Input: part model. Units: mm. Frame: model coordinates. Face numbers are marked on the shaded views. A direction names the side the tool comes from. Coordinates: 2 decimals unless noted, no trailing zeros. Loops run counter-clockwise (first coordinate to the right, second up) from the corner with the lowest first, then second, coordinate; pieces in that order, holes last. Notation, with made-up numbers: (-37.75, -30) -> (5.25, -30) arc R7 ccw to (5.25, -23) -> close; hole circle Ø2 at (53, 32). An arc over 180 degrees is marked (long way). Answer as a JSON object with one key per item and string values.
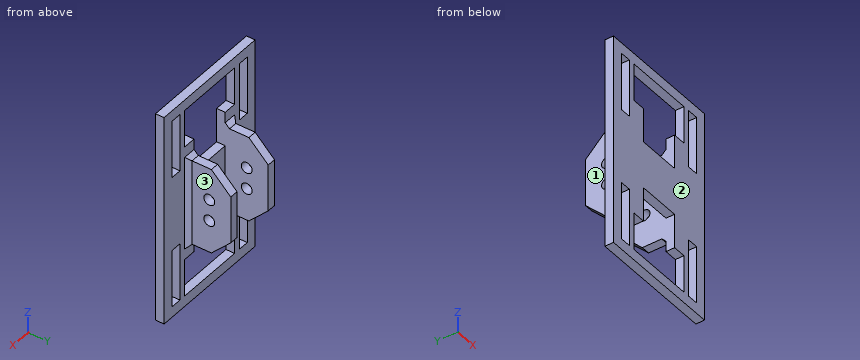
from build123d import *

# Parameters (mm, degrees)
SKETCH1_W           = 58.28
SKETCH1_H           = 99
SKETCH1_W_2         = 5.14
SKETCH1_H_2         = 27
BOSS_EXTRUDE1_DEPTH = 4
SKETCH2_W           = 4
SKETCH2_H           = 40
BOSS_EXTRUDE2_DEPTH = 20
CUT_EXTRUDE1_REACH  = 108.175
SKETCH3_R           = 2.55
CHAMFER1_SIZE       = 2
CUT_EXTRUDE2_REACH  = 108.175
CUT_EXTRUDE3_DEPTH  = 4


with BuildPart() as part:
    # Sketch1 → Boss-Extrude1 (new body)
    with BuildSketch(Plane(origin=(0, 0, 0), x_dir=(1, 0, 0), z_dir=(0, 1, 0))):
        with Locations((24.14, 44.5)):
            Rectangle(SKETCH1_W, SKETCH1_H)
        with Locations((2.57, 75.5)):
            Rectangle(SKETCH1_W_2, SKETCH1_H_2, mode=Mode.SUBTRACT)
        with Locations((45.71, 75.5)):
            Rectangle(SKETCH1_W_2, SKETCH1_H_2, mode=Mode.SUBTRACT)
        with Locations((2.57, 13.5)):
            Rectangle(SKETCH1_W_2, SKETCH1_H_2, mode=Mode.SUBTRACT)
        with Locations((45.71, 13.5)):
            Rectangle(SKETCH1_W_2, SKETCH1_H_2, mode=Mode.SUBTRACT)
    extrude(amount=BOSS_EXTRUDE1_DEPTH)

    # Sketch2 → Boss-Extrude2 (add)
    with BuildSketch(Plane(origin=(0, 4, 0), x_dir=(1, 0, 0), z_dir=(0, 1, 0))):
        with Locations((12.14, 44.5)):
            Rectangle(SKETCH2_W, SKETCH2_H)
        with Locations((36.14, 44.5)):
            Rectangle(SKETCH2_W, SKETCH2_H)
    extrude(amount=BOSS_EXTRUDE2_DEPTH)

    # Cut-Extrude1: up to this face of the body (flat: up to its plane)
    cut_extrude1_end = Plane(part.part.faces().sort_by_distance((10.14, 14, -44.5))[0])
    # Sketch3 → Cut-Extrude1 (cut, up to the picked face)
    with BuildSketch(Plane(origin=(38.14, 0, 0), x_dir=(0, 0, -1), z_dir=(1, 0, 0)), mode=Mode.PRIVATE) as cut_extrude1_sk1:
        with Locations((39.5, 14)):
            Circle(SKETCH3_R)
    cut_extrude1_tool1 = split(extrude(cut_extrude1_sk1.sketch, amount=-CUT_EXTRUDE1_REACH, mode=Mode.PRIVATE), bisect_by=cut_extrude1_end, keep=Keep.BOTH, mode=Mode.PRIVATE)
    # Sketch3 → Cut-Extrude1 (cut, up to the picked face)
    with BuildSketch(Plane(origin=(38.14, 0, 0), x_dir=(0, 0, -1), z_dir=(1, 0, 0)), mode=Mode.PRIVATE) as cut_extrude1_sk2:
        with Locations((49.5, 14)):
            Circle(SKETCH3_R)
    cut_extrude1_tool2 = split(extrude(cut_extrude1_sk2.sketch, amount=-CUT_EXTRUDE1_REACH, mode=Mode.PRIVATE), bisect_by=cut_extrude1_end, keep=Keep.BOTH, mode=Mode.PRIVATE)
    add(cut_extrude1_tool1.solids().sort_by(Axis((38.14, 14, -39.5), (-1, 0, 0)))[0], mode=Mode.SUBTRACT)
    add(cut_extrude1_tool2.solids().sort_by(Axis((38.14, 14, -49.5), (-1, 0, 0)))[0], mode=Mode.SUBTRACT)

    # Chamfer1
    chamfer1_edges = [part.edges().sort_by_distance(p)[0] for p in [
        (12.14, 4, -64.5),
        (10.14, 4, -44.5),
        (12.14, 4, -24.5),
        (36.14, 4, -24.5),
        (38.14, 4, -44.5),
        (36.14, 4, -64.5),
    ]]
    chamfer(chamfer1_edges, length=CHAMFER1_SIZE)

    # Cut-Extrude2: up to this face of the body (flat: up to its plane)
    cut_extrude2_end = Plane(part.part.faces().sort_by_distance((38.14, 15.060158725, -44.5))[0])
    # Sketch4 → Cut-Extrude2 (cut, up to the picked face)
    with BuildSketch(Plane.ZY.offset(-10.14), mode=Mode.PRIVATE) as cut_extrude2_sk1:
        Polygon((-55.5, 24), (-64.5, 15), (-64.5, 24), align=None)
    cut_extrude2_tool1 = split(extrude(cut_extrude2_sk1.sketch, amount=-CUT_EXTRUDE2_REACH, mode=Mode.PRIVATE), bisect_by=cut_extrude2_end, keep=Keep.BOTH, mode=Mode.PRIVATE)
    # Sketch4 → Cut-Extrude2 (cut, up to the picked face)
    with BuildSketch(Plane.ZY.offset(-10.14), mode=Mode.PRIVATE) as cut_extrude2_sk2:
        Polygon((-33.5, 24), (-24.5, 15), (-24.5, 24), align=None)
    cut_extrude2_tool2 = split(extrude(cut_extrude2_sk2.sketch, amount=-CUT_EXTRUDE2_REACH, mode=Mode.PRIVATE), bisect_by=cut_extrude2_end, keep=Keep.BOTH, mode=Mode.PRIVATE)
    add(cut_extrude2_tool1.solids().sort_by(Axis((10.14, 21, -61.5), (1, 0, 0)))[0], mode=Mode.SUBTRACT)
    add(cut_extrude2_tool2.solids().sort_by(Axis((10.14, 21, -27.5), (1, 0, 0)))[0], mode=Mode.SUBTRACT)

    # Sketch5 → Cut-Extrude3 (cut)
    with BuildSketch(Plane(origin=(0, 4, 0), x_dir=(1, 0, 0), z_dir=(0, 1, 0))):
        Polygon((8.14, 89), (40.14, 89), (40.14, 71.5), (34.14, 71.5), (34.14, 55.5), (14.14, 55.5), (14.14, 71.5), (8.14, 71.5), align=None)
        Polygon((8.14, 0), (40.14, 0), (40.14, 17.5), (34.14, 17.5), (34.14, 33.5), (14.14, 33.5), (14.14, 17.5), (8.14, 17.5), align=None)
    extrude(amount=-CUT_EXTRUDE3_DEPTH, mode=Mode.SUBTRACT)


solid = part.part
1. Access query for the marked faces 1, 2 and 3. Directions: +Z, -Z, +X, -X, +Y, -Y. A direction counts if a zero-diameter tool reaches every point of the face in a straight line with its end or side. Return the directions, or none.
Reply:
{"face 1": "+Z, -Z, -X, +Y", "face 2": "+Z, -Z, +X, -X, -Y", "face 3": "+Z, -Z, +X, +Y"}
2. Section query D-D (y = 18.75). Return loops of the section in (x, z), plus the area to 3 significant figures.
Reply:
{"outline": "(10.14, -60.75) -> (14.14, -60.75) -> (14.14, -28.25) -> (10.14, -28.25) -> close; (34.14, -60.75) -> (38.14, -60.75) -> (38.14, -28.25) -> (34.14, -28.25) -> close", "area": "260 mm2"}
3. Pin query (flat end, axial travel): P1, Ø1, axis at x = 36.5, z = -24.5, coming from the +Y side; P2, Ø3, axis at y = 12.5, z = -48, coming from the -X side; P3, Ø10, axis at x = 12, z = -65.5, coming from the +Y side. Return the tip coordinate at first contact, or that it passes through.
Reply:
{"P1": "stops at y = 15.5", "P2": "stops at x = 10.14", "P3": "stops at y = 19"}
4. Line query: line 1 along X through (y, z) = (3.25, -20); line 2 along X through (y, z) = (9, -41); line 3 along X through (y, z) = (3.75, -8). Output: solid intervals per line, ascending.
Reply:
{"line 1": "x = -5 to 0, 5.14 to 14.14, 34.14 to 43.14, 48.28 to 53.28", "line 2": "x = 10.14 to 14.14, 34.14 to 38.14", "line 3": "x = -5 to 0, 5.14 to 8.14, 40.14 to 43.14, 48.28 to 53.28"}
5. Section query B-B (y = 14). Return loops of the section in (x, z), plus the area to 3 significant figures.
Reply:
{"outline": "(10.14, -64.5) -> (14.14, -64.5) -> (14.14, -52.05) -> (10.14, -52.05) -> close; (10.14, -46.95) -> (14.14, -46.95) -> (14.14, -42.05) -> (10.14, -42.05) -> close; (10.14, -36.95) -> (14.14, -36.95) -> (14.14, -24.5) -> (10.14, -24.5) -> close; (34.14, -64.5) -> (38.14, -64.5) -> (38.14, -52.05) -> (34.14, -52.05) -> close; (34.14, -46.95) -> (38.14, -46.95) -> (38.14, -42.05) -> (34.14, -42.05) -> close; (34.14, -36.95) -> (38.14, -36.95) -> (38.14, -24.5) -> (34.14, -24.5) -> close", "area": "238 mm2"}
6. Section query A-A (x = 29.5). Return loops of the section in (y, z).
Reply:
{"outline": "(0, -94) -> (4, -94) -> (4, -89) -> (0, -89) -> close; (0, -55.5) -> (4, -55.5) -> (4, -33.5) -> (0, -33.5) -> close; (0, 0) -> (4, 0) -> (4, 5) -> (0, 5) -> close"}
7. Section query C-C (z = -69). Return loops of the section in (x, y), plus the area to 3 significant figures.
Reply:
{"outline": "(-5, 0) -> (0, 0) -> (0, 4) -> (-5, 4) -> close; (5.14, 0) -> (14.14, 0) -> (14.14, 4) -> (5.14, 4) -> close; (34.14, 0) -> (43.14, 0) -> (43.14, 4) -> (34.14, 4) -> close; (48.28, 0) -> (53.28, 0) -> (53.28, 4) -> (48.28, 4) -> close", "area": "112 mm2"}
